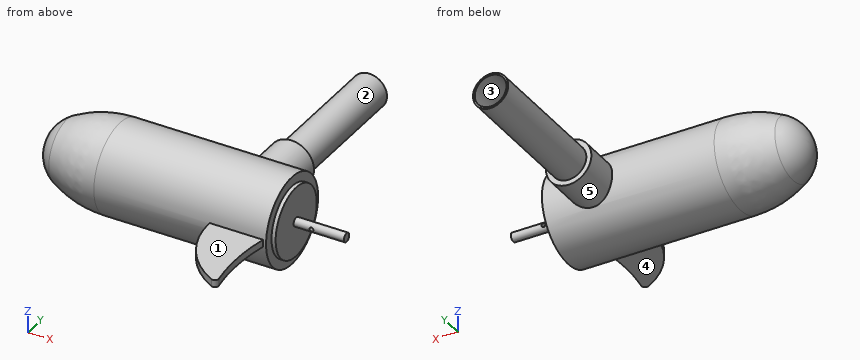
from build123d import *

# Parameters (mm, degrees)
SKETCH2_R                = 12.573
SKETCH2_R_2              = 11.303
BOSS_EXTRUDE1_DEPTH      = 635
SKETCH4_W                = 38.1
SKETCH4_H                = 6.35
BOSS_EXTRUDE3_DEPTH      = 2.54
BOSS_EXTRUDE3_DEPTH_BACK = 2.54
FILLET1_R                = 2.54
SKETCH5_R                = 16.1925
BOSS_EXTRUDE4_DEPTH      = 57.15
SKETCH6_W                = 25.146
SKETCH6_H                = 355.6
CUT_EXTRUDE1_DEPTH       = 32.7500001
CUT_EXTRUDE1_DEPTH_BACK  = 32.7500001
SKETCH7_R                = 36.277914584
CUT_EXTRUDE2_DEPTH       = 4.15798
SKETCH8_R                = 25.0825
BOSS_EXTRUDE5_DEPTH      = 2.9464
SKETCH9_R                = 3.175
BOSS_EXTRUDE6_DEPTH      = 35.941
SKETCH10_R               = 1.4224
CUT_EXTRUDE3_DEPTH       = 280.4
CUT_EXTRUDE3_DEPTH_BACK  = 88.034563121
SKETCH11_R               = 17.161337021
CUT_EXTRUDE4_DEPTH       = 127


with BuildPart() as part:
    # Sketch1 one side → Revolve1 (revolve)
    with BuildSketch(Plane.XY):
        with BuildLine():
            Line((38.1, 31.75), (-88.9, 31.75))
            ThreePointArc((-88.9, 31.75), (-108.34073355, 29.331909563), (-126.596722124, 22.225))
            ThreePointArc((-126.596722124, 22.225), (-136.180319261, 12.90006314), (-139.7, 0))
            Line((-139.7, 0), (-88.9, 0))
            Line((-88.9, 0), (38.1, 0))
            Line((38.1, 0), (38.1, 31.75))
        make_face()
    revolve(axis=Axis((0, 0, 0), (-1, 0, 0)))

    # Sketch2 → Boss-Extrude1 (add)
    with BuildSketch(Plane(origin=(0, 0, 0), x_dir=(1, 0, 0), z_dir=(0, 1, 0))):
        Circle(SKETCH2_R)
        Circle(SKETCH2_R_2, mode=Mode.SUBTRACT)
    extrude(amount=BOSS_EXTRUDE1_DEPTH)

    # Sketch4 → Boss-Extrude3 (add, two sides)
    with BuildSketch(Plane.XY) as boss_extrude3_sk:
        with BuildLine():
            ThreePointArc((31.75, -31.75), (28.726104864, -60.325), (31.75, -88.9))
            ThreePointArc((31.75, -88.9), (4.048186152, -66.092875899), (-6.35, -31.75))
            Line((-6.35, -31.75), (31.75, -31.75))
        make_face()
        with Locations((12.7, -28.575)):
            Rectangle(SKETCH4_W, SKETCH4_H)
    extrude(amount=BOSS_EXTRUDE3_DEPTH)
    extrude(boss_extrude3_sk.sketch, amount=-BOSS_EXTRUDE3_DEPTH_BACK)

    # Fillet1
    fillet1_edges = [part.edges().sort_by_distance(p)[0] for p in [
        (31.75, -88.9, 0),
    ]]
    fillet(fillet1_edges, radius=FILLET1_R)

    # Sketch5 → Boss-Extrude4 (add)
    with BuildSketch(Plane(origin=(0, 0, 0), x_dir=(1, 0, 0), z_dir=(0, 1, 0))):
        Circle(SKETCH5_R)
    extrude(amount=BOSS_EXTRUDE4_DEPTH)

    # Sketch6 → Cut-Extrude1 (cut, two sides)
    with BuildSketch(Plane.XY) as cut_extrude1_sk:
        with Locations((0, 457.2)):
            Rectangle(SKETCH6_W, SKETCH6_H)
    extrude(amount=CUT_EXTRUDE1_DEPTH, mode=Mode.SUBTRACT)
    extrude(cut_extrude1_sk.sketch, amount=-CUT_EXTRUDE1_DEPTH_BACK, mode=Mode.SUBTRACT)

    # Sketch7 → Cut-Extrude2 (cut)
    with BuildSketch(Plane(origin=(38.1, 0, 0), x_dir=(0, 0, -1), z_dir=(1, 0, 0))):
        Circle(SKETCH7_R)
    extrude(amount=-CUT_EXTRUDE2_DEPTH, mode=Mode.SUBTRACT)

    # Sketch8 → Boss-Extrude5 (add)
    with BuildSketch(Plane(origin=(33.94202, 0, 0), x_dir=(0, 0, -1), z_dir=(1, 0, 0))):
        Circle(SKETCH8_R)
    extrude(amount=BOSS_EXTRUDE5_DEPTH)

    # Sketch9 → Boss-Extrude6 (add)
    with BuildSketch(Plane(origin=(36.88842, 0, 0), x_dir=(0, 0, -1), z_dir=(1, 0, 0))):
        Circle(SKETCH9_R)
    extrude(amount=BOSS_EXTRUDE6_DEPTH)

    # Sketch10 → Cut-Extrude3 (cut, two sides)
    with BuildSketch(Plane(origin=(0, 0, 0), x_dir=(1, 0, 0), z_dir=(0, 1, 0))) as cut_extrude3_sk:
        with Locations((49.58842, 0)):
            Circle(SKETCH10_R)
    extrude(amount=CUT_EXTRUDE3_DEPTH, mode=Mode.SUBTRACT)
    extrude(cut_extrude3_sk.sketch, amount=-CUT_EXTRUDE3_DEPTH_BACK, mode=Mode.SUBTRACT)

    # Sketch11 → Cut-Extrude4 (cut)
    with BuildSketch(Plane(origin=(0, 279.4, 0), x_dir=(1, 0, 0), z_dir=(0, 1, 0))):
        Circle(SKETCH11_R)
    extrude(amount=-CUT_EXTRUDE4_DEPTH, mode=Mode.SUBTRACT)


solid = part.part
Design review of the part built by this model. Coordinates are the model's own, in mm. Face numbers are marked on the shaded views. A direction names the side the tool comes from. Give positions to 0.01 mm unless a question says otherwise; leave off trailing zeros. Order: outer loops, then holes, each group sorted by start corner. A loop starts at its lowest first (then second) coordinate and runs counter-clockwise, first axis right, second up. Notation, with made-up numbers: (-19, 12) - (-1, 12) arc R34 ccw to (-1, 46) - close; hole circle Ø7 at (-4.75, 77). An arc over 180 degrees is marked (long way). Use CSV: the item, a comma, the result in double quotes. Start each with the question number.
Q1. Take a section at B-B (y = 41). State the section outline as (x, z) points (1 decimal).
Q2. Draft analysis for pull direction X (two halves, no side actions). For the marked faces 3, 4 and 5, state which applies: pulls with the +X half, pulls with the -X half, needs draft (parallel to the pull), parting line crosses it, or undercut.
Q3. For line 1 (Z direction, x = 0, y = 89); line 2 (X direction, y = -0.85, z = 0); line 3 (X direction, y = 77.5, z = -4), list the stretches that pass through material, from the lowest coordinate up.
Q4. Take a section at D-D (y = -37.5). State the section outline as (x, z) points, and give its area (3 significant figures).
Q5. Take a section at C-C (x = 55.5). State the section outline as (y, z) points (3 decimals), and give its area (3 significant figures).
Q6. Take a section at A-A (x = 0). State the section outline as (y, z) points, and give its area (3 significant figures).
Q7. For P1, Ø2, axis at x = -61.5, z = -17, coming from the +Y side; P2, Ø6, axis at y = -33, z = -7, coming from the +X side; P3, Ø4, axis at x = 25, z = -23, coming from the +Y side; P4, Ø2.5, axis at x = 49.59, z = 0, coming from the -Y side, all flat-tipped, find the tip position at first contact; note any pin that passes through.
Q8. Machinability: for the marked faces 1 and 2, which of the approach directions +Z, -Z, +X, -X, +Y, -Y give a long, thin tool a straight path to every point of the face, cutting with its end or side? Answer none if there is none.
Calculated:
1,outline,"circle Ø32.4 at (0, 0)"
2,face 3,"undercut"
2,face 4,"needs draft"
2,face 5,"parting line crosses it"
3,line 1,"z = -12.57 to -11.3, 11.3 to 12.57"
3,line 2,"x = -139.69 to 48.17, 51.01 to 72.83"
3,line 3,"x = -11.92 to -10.57, 10.57 to 11.92"
4,outline,"(-6.08, -2.54) - (30.65, -2.54) - (30.65, 2.54) - (-6.08, 2.54) - close"
4,area,"187 mm²"
5,outline,"circle Ø6.35 at (0, 0)"
5,area,"31.7 mm²"
6,outline,"(-59.06, -2.54) - (-31.65, -2.54) arc R31.75 ccw to (27.31, -16.19) - (57.15, -16.19) - (57.15, -12.57) - (152.4, -12.57) - (152.4, -11.3) - (57.15, -11.3) - (57.15, 11.3) - (152.4, 11.3) - (152.4, 12.57) - (57.15, 12.57) - (57.15, 16.19) - (27.31, 16.19) arc R31.75 ccw to (-31.65, 2.54) - (-59.06, 2.54) - close"
6,area,"4,420 mm²"
7,P1,"stops at y = 27.42"
7,P2,"stops at x = 33.94"
7,P3,"stops at y = 23.81"
7,P4,"passes through"
8,face 1,"+Z, +X, -X, -Y"
8,face 2,"+Y"
